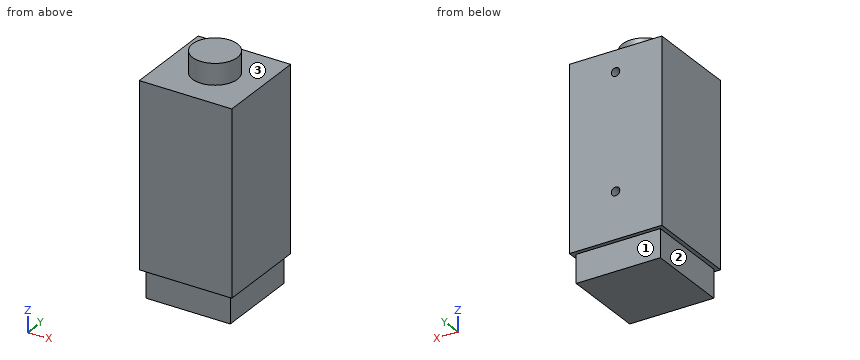
```python
from build123d import *

# Parameters (mm, degrees)
ESBO_O1_W                = 33
ESBO_O1_H                = 33
RESSALTO_EXTRUS_O1_DEPTH = 65
ESBO_O2_W                = 30
ESBO_O2_H                = 30
RESSALTO_EXTRUS_O2_DEPTH = 10
ESBO_O3_R                = 8
RESSALTO_EXTRUS_O3_DEPTH = 7.5
ESBO_O4_R                = 1.5
CORTE_EXTRUS_O1_DEPTH    = 7.5


with BuildPart() as part:
    # Esboço1 → Ressalto-extrusão1 (new body)
    with BuildSketch(Plane.XY):
        Rectangle(ESBO_O1_W, ESBO_O1_H)
    extrude(amount=RESSALTO_EXTRUS_O1_DEPTH)

    # Esboço2 → Ressalto-extrusão2 (add)
    with BuildSketch(Plane(origin=(0, 0, 0), x_dir=(-1, 0, 0), z_dir=(0, 0, -1))):
        Rectangle(ESBO_O2_W, ESBO_O2_H)
    extrude(amount=RESSALTO_EXTRUS_O2_DEPTH)

    # Esboço3 → Ressalto-extrusão3 (add)
    with BuildSketch(Plane.XY.offset(65)):
        Circle(ESBO_O3_R)
    extrude(amount=RESSALTO_EXTRUS_O3_DEPTH)

    # Esboço4 → Corte-extrusão1 (cut)
    with BuildSketch(Plane(origin=(0, 16.5, 0), x_dir=(1, 0, 0), z_dir=(0, 1, 0))):
        with Locations((0, -16.5)):
            Circle(ESBO_O4_R)
        with Locations((0, -57.5)):
            Circle(ESBO_O4_R)
    extrude(amount=-CORTE_EXTRUS_O1_DEPTH, mode=Mode.SUBTRACT)


solid = part.part
```
For this review, take the finished solid that the model builds, in its own axes (mm). Face numbers are marked on the shaded views. A direction names the side the tool comes from. Round coordinates to 2 decimals unless told otherwise and drop trailing zeros. Order: outer loops, then holes, each group sorted by start corner. A loop starts at its lowest first (then second) coordinate and runs counter-clockwise, first axis right, second up.
Q1. Wall thickness on line 1 (Z direction, x = 0, y = 12.25); line 2 (X direction, y = 12.75, z = 57.5); line 3 (Z direction, x = 4.5, y = 12): over which ranges is each line inside the solid? List them lowest first.
Findings below:
line 1: z = -10 to 15, 18 to 56, 59 to 65
line 2: x = -16.5 to -1.5, 1.5 to 16.5
line 3: z = -10 to 65
Q2. Insertion check: P1, Ø8, axis at x = -4.5, z = -7, coming from the +Y side; P2, Ø3, axis at y = -4.5, z = -5, coming from the -X side; P3, Ø8, axis at y = -3.5, z = -7, coming from the +X side. Each pin has a flat end and moves straight along its axis. Give the tip position at first contact, or say it passes through.
Findings below:
P1: stops at y = 15
P2: stops at x = -15
P3: stops at x = 15
Q3. Machinability: for the marked faces 1, 2 and 3, which of the approach directions +Z, -Z, +X, -X, +Y, -Y give a long, thin tool a straight path to every point of the face, cutting with its end or side? Answer none if there is none.
Findings below:
face 1: -Z, +X, -X, +Y
face 2: -Z, -X, +Y, -Y
face 3: +Z
Q4. We need section B-B, the plane x = 0. Give the boundary of the cut face in (y, z), plus the area to 3 significant figures.
Findings below:
outline: (-16.5, 0) - (-15, 0) - (-15, -10) - (15, -10) - (15, 0) - (16.5, 0) - (16.5, 15) - (9, 15) - (9, 18) - (16.5, 18) - (16.5, 56) - (9, 56) - (9, 59) - (16.5, 59) - (16.5, 65) - (8, 65) - (8, 72.5) - (-8, 72.5) - (-8, 65) - (-16.5, 65) - close
area: 2,520 mm2
Q5. We need section A-A, the plane y = 13. Give the boundary of the cut face in (x, z).
Findings below:
outline: (-16.5, 0) - (-15, 0) - (-15, -10) - (15, -10) - (15, 0) - (16.5, 0) - (16.5, 65) - (-16.5, 65) - close; hole circle Ø3 at (0, 16.5); hole circle Ø3 at (0, 57.5)
Q6. We need section C-C, the plane y = -12. Give the boundary of the cut face in (x, z).
Findings below:
outline: (-16.5, 0) - (-15, 0) - (-15, -10) - (15, -10) - (15, 0) - (16.5, 0) - (16.5, 65) - (-16.5, 65) - close
Q7. We need section D-D, the plane z = 57.5. Give the boundary of the cut face in (x, y).
Findings below:
outline: (-16.5, -16.5) - (16.5, -16.5) - (16.5, 16.5) - (1.5, 16.5) - (1.5, 9) - (-1.5, 9) - (-1.5, 16.5) - (-16.5, 16.5) - close
